Input: dimensioned drawing with shaded views. Units: mm. Origin: part minimum x, y, z. A direction names the side the tool comes from. Give positions to 0.01 mm unless a question says otherwise; leave off trailing zeros. Order: outer loops, then holes, each group sorted by start corner. A loop starts at its lowest first (then second) coordinate and runs counter-clockwise, first axis right, second up. Notation, with made-up numbers: (61, 5) - (109, 5) arc R26 cw to (109, 29) - close; hole circle Ø9 at (-17.5, 19.25). An arc over 180 degrees is marked (long way). Use a Markdown table: item, result.
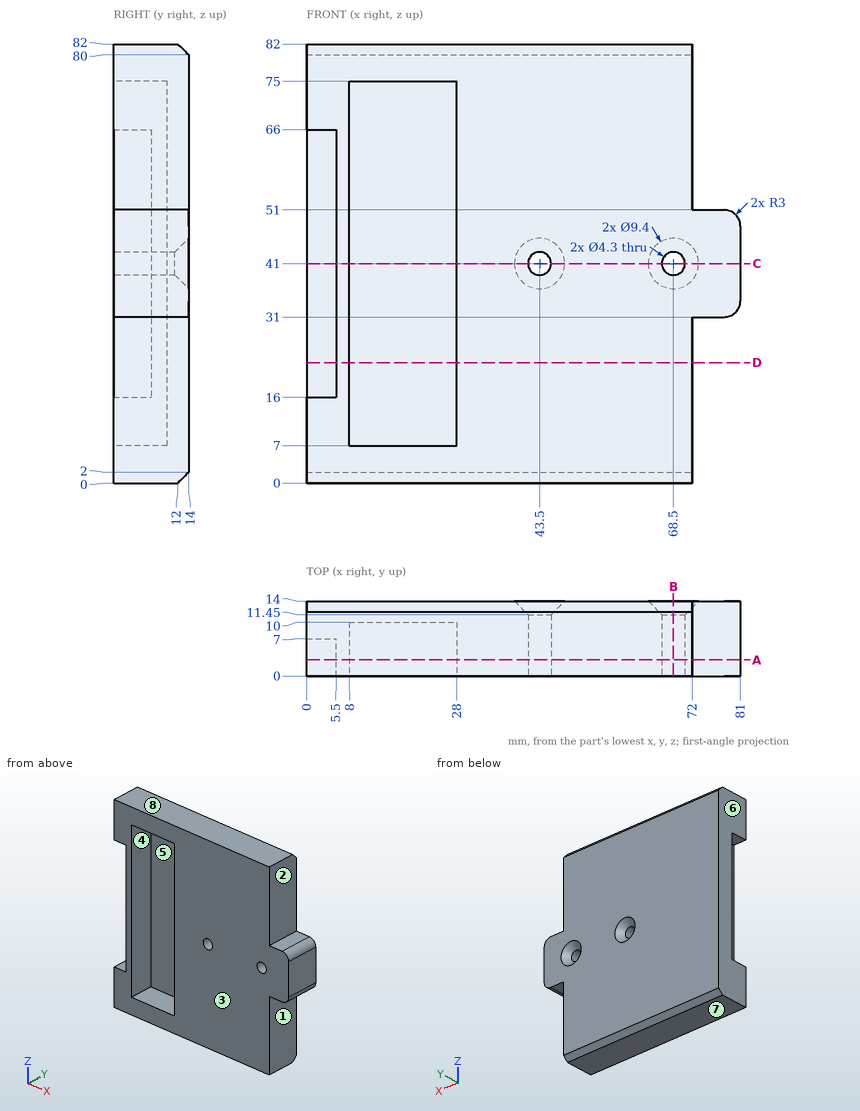
1. Section query B-B (x = 68.5). Return loops of the section in (y, z).
Response:
| item | result |
|---|---|
| outline | (0, 0) - (12, 0) - (14, 2) - (14, 36.3) - (11.45, 38.85) - (0, 38.85) - close; (0, 43.15) - (11.45, 43.15) - (14, 45.7) - (14, 80) - (12, 82) - (0, 82) - close |
2. Section query C-C (z = 41). Return loops of the section in (x, y), then the cut area to 3 significant figures.
Response:
| item | result |
|---|---|
| outline | (0, 7) - (5.5, 7) - (5.5, 0) - (8, 0) - (8, 10) - (28, 10) - (28, 0) - (41.35, 0) - (41.35, 11.45) - (38.8, 14) - (0, 14) - close; (45.65, 0) - (66.35, 0) - (66.35, 11.45) - (63.8, 14) - (48.2, 14) - (45.65, 11.45) - close; (70.65, 0) - (81, 0) - (81, 14) - (73.2, 14) - (70.65, 11.45) - close |
| area | 762 mm^2 |
3. Material intervals for line 1 along X through (y, z) = (9.25, 41); line 2 along X through (y, z) = (3.75, 41); line 3 along Z through (x, y) = (68.5, 3), sorted ascending.
Response:
| item | result |
|---|---|
| line 1 | x = 0 to 8, 28 to 41.35, 45.65 to 66.35, 70.65 to 81 |
| line 2 | x = 5.5 to 8, 28 to 41.35, 45.65 to 66.35, 70.65 to 81 |
| line 3 | z = 0 to 38.85, 43.15 to 82 |
4. Mould query, pull axis Z, two halves, no side actions, for the marked faces 5, 6, 7 and 8. Classes: pulls with the +Z half, pulls with the -Z half, needs draft (parallel to the pull), parting line crosses it, or undercut.
Response:
| item | result |
|---|---|
| face 5 | undercut |
| face 6 | needs draft |
| face 7 | pulls with the -Z half |
| face 8 | pulls with the +Z half |
5. Section query A-A (y = 3). Return loops of the section in (x, z), then the cut area to 3 significant figures.
Response:
| item | result |
|---|---|
| outline | (0, 0) - (72, 0) - (72, 31) - (78, 31) arc R3 ccw to (81, 34) - (81, 48) arc R3 ccw to (78, 51) - (72, 51) - (72, 82) - (0, 82) - (0, 66) - (5.5, 66) - (5.5, 16) - (0, 16) - close; hole (8, 7) - (28, 7) - (28, 75) - (8, 75) - close; hole circle Ø4.3 at (43.5, 41); hole circle Ø4.3 at (68.5, 41) |
| area | 4,420 mm^2 |
6. Set-up query: the marked faces 1, 2, 3 and 4. Return all of +Z, -Z, +X, -X, +Y, -Y with unobstructed straight access to the full face (end or side cutting, diameter ignored); none if empty.
Response:
| item | result |
|---|---|
| face 1 | -Z, +X, +Y, -Y |
| face 2 | +Z, +X, +Y, -Y |
| face 3 | +Z, -Z, +X, -X, -Y |
| face 4 | -Y |
7. Section query D-D (z = 22.5). Return loops of the section in (x, y), then the cut area to 4 significant figures.
Response:
| item | result |
|---|---|
| outline | (0, 7) - (5.5, 7) - (5.5, 0) - (8, 0) - (8, 10) - (28, 10) - (28, 0) - (72, 0) - (72, 14) - (0, 14) - close |
| area | 769.5 mm^2 |
8. Pin query (flat end, axial travel): pin 1 (4 mm diameter, centred on y = 9.5, z = 19, fed in from +X); pin 2 (5.5 mm diameter, centred on x = 43.5, z = 41, fed in from +Y); pin 3 (1 mm diameter, centred on x = 54.5, z = 58.5, fed in from -Y); pin 4 (1.6 mm diameter, centred on x = 3.5, z = 47, fed in from -Y). Return the tip coordinate at first contact, or that it passes through.
Response:
| item | result |
|---|---|
| pin 1 | stops at x = 72 |
| pin 2 | stops at y = 12.05 |
| pin 3 | stops at y = 0 |
| pin 4 | stops at y = 7 |
